Check sheet for the modelled part. Datum: model origin and axes. Units: mm. Round coordinates to 2 decimals unless told otherwise and drop trailing zeros. Loops run counter-clockwise (first coordinate to the right, second up) from the corner with the lowest first, then second, coordinate; pieces in that order, holes last. Notation, with made-up numbers: M 6.5,82.25 L 16.5,82.25 A20 ccw 16.5,101.25 Z; hole C -9,18.5 d11. An arc over 180 degrees is marked long. One line per question, with ' | ' between items. Start each with the question number.
(1) Go/stop test with flat-tipped pins: P1, Ø2, axis at x = -1, y = 8.5, coming from the +Z side; P2, Ø1.5, axis at x = 9, z = -9, coming from the +Y side; P3, Ø4, axis at y = -7.5, z = -14.5, coming from the +X side. Record where each tip stops, or that it passes through.
(2) Thickness scan on probe 1 along Y at (x, z) = (0, -5.25); probe 2 along Y at (x, z) = (3.75, -2); probe 3 along Z at (x, y) = (-1.75, 7). Record the ranges inside material, lowest first. Write a range as [from, to].
(3) Section check D-D (z = -1.25). Record the boundary of the cut face in (x, y), and give its area (3 significant figures).
(4) Section check B-B (z = -13.25). Record the boundary of the cut face in (x, y), and give its area (3 significant figures).
(5) Draft check along Y on faces 1 (the face through (-1.5, 11.4, -9.4)), 2 (the face through (9.252, 2.914, -8.48)), 3 (the face through (0, 0, -19)). Enter one of: +Y half, -Y half, draft (parallel to the pull), parting line (faces both ways), or undercut.
(6) Section check A-A (y = 0). Record the boundary of the cut face in (x, z), and give its area (3 significant figures).
```python
from build123d import *

# Parameters (mm, degrees)
F0_R     = 11.5
F1_DEPTH = 19
F2_T     = -1.8


# Not quite as in the source:
# - a fillet or chamfer that OpenCascade refuses, or shapes differently, is made with other operations: its cross-section is extruded or revolved along the edge and cut away or added


with BuildPart() as f1:
    # F0 (on Top) → F1 (new body)
    with BuildSketch(Plane.XY):
        Circle(F0_R)
    extrude(amount=-F1_DEPTH)

    # F2
    f2_openings = [f1.faces().sort_by_distance(p)[0] for p in [
        (0, 0, 0),
    ]]
    offset(amount=F2_T, openings=f2_openings)

    # F3: fillet of radius 2 on 2 edges, made by hand

    # F3_s1 → F3_t2 (revolve, cut)
    with BuildSketch(Plane.XZ):
        with BuildLine():
            ThreePointArc((11.5, -17), (10.9142135624, -18.4142135624), (9.5, -19))
            Line((9.5, -19), (11.5, -19))
            Line((11.5, -19), (11.5, -17))
        make_face()
    revolve(axis=Axis((0, 0, -19), (0, 0, 1)), mode=Mode.SUBTRACT)

    # F3_s3 → F3_t4 (revolve, cut)
    with BuildSketch(Plane.XZ):
        with BuildLine():
            ThreePointArc((11.5, -1.9899748742), (10.9832396974, -0.6483340877), (9.7, 0))
            Line((9.7, 0), (11.5, 0))
            Line((11.5, 0), (11.5, -1.9899748742))
        make_face()
    revolve(axis=Axis((0, 0, 0), (0, 0, 1)), mode=Mode.SUBTRACT)


solid = f1.part
```
The answers:
1) P1: z = -17.2 | P2: y = 8.01 | P3: x = 10.1
2) probe 1: [-11.5, -9.7], [9.7, 11.5] | probe 2: [-10.87, -8.95], [8.95, 10.87] | probe 3: [-19, -17.2]
3) outline: C 0,0 d22.72; hole C 0,0 d19.4 | area: 110 mm²
4) outline: C 0,0 d23; hole C 0,0 d19.4 | area: 120 mm²
5) face 1: parting line | face 2: undercut | face 3: draft
6) outline: M -11.5,-17 A2 ccw -9.5,-19 L 9.5,-19 A2 ccw 11.5,-17 L 11.5,-1.99 A2 ccw 9.7,0 L 9.7,-17.2 L -9.7,-17.2 L -9.7,0 A2 ccw -11.5,-1.99 Z | area: 99.9 mm²
